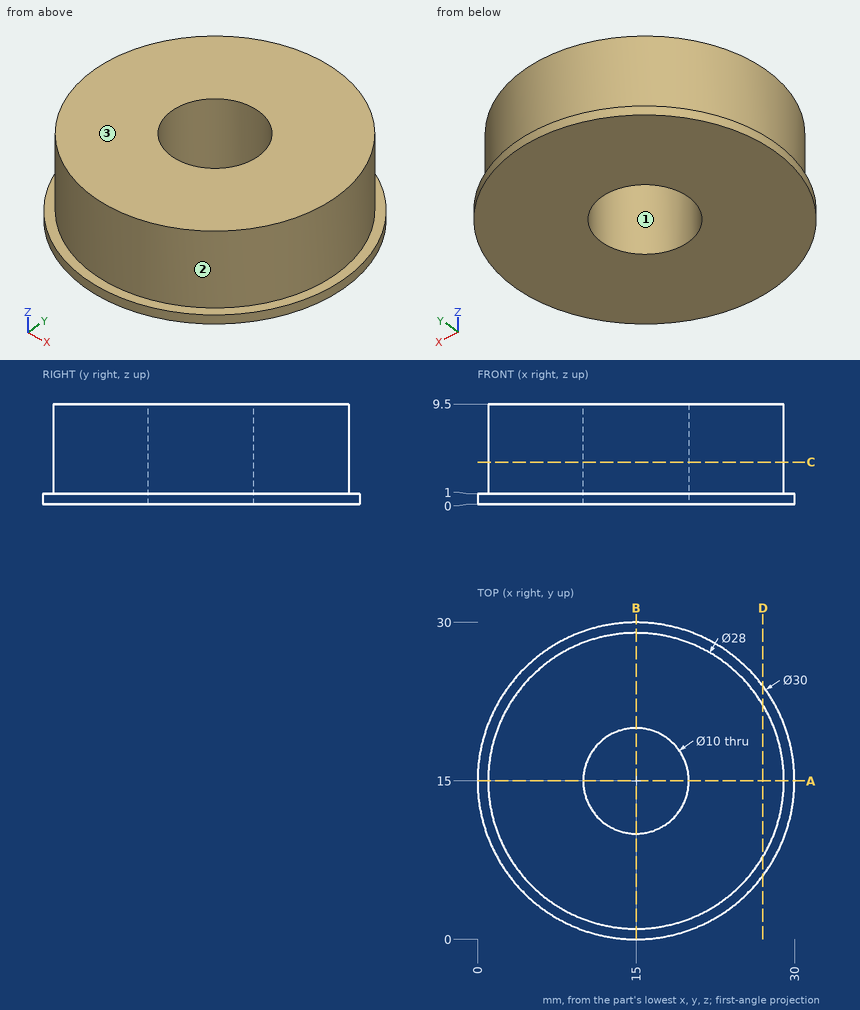
Geometry check sheet. Reference: drawing and pictorial views, mm from the part's lowest x, y, z. Coordinates: 2 decimals unless noted, no trailing zeros. Order: outer loops, then holes, each group sorted by start corner. A loop starts at its lowest first (then second) coordinate and runs counter-clockwise, first axis right, second up. Notation, with made-up numbers: (84.5, -38.5) -> (117.5, -38.5) arc R20 cw to (117.5, -32.5) -> close; hole circle Ø8 at (8.25, 50.25). An arc over 180 degrees is marked (long way). Write item = value, one per line. Start each with the question number.
1) Go/stop test with flat-tipped pins: P1, Ø2, axis at y = 8.5, z = 5.5, coming from the +X side; P2, Ø5, axis at x = 23.5, y = 16.5, coming from the -Z side; P3, Ø1, axis at x = 13.5, z = 2, coming from the +Y side; P4, Ø3, axis at y = 12.5, z = 5, coming from the -X side. Record where each tip stops, or that it passes through.
2) Mould release check, pull along X, two halves, no side actions. Record for the marked faces 1, 2 and 3: +X half, -X half, draft (parallel to the pull), parting line (faces both ways), or undercut.
3) Cross-section at A-A (y = 15). Enter the section's corners in (x, z), then the cut area to 3 significant figures.
4) Cross-section at C-C (z = 4). Enter the section's corners in (x, y).
5) Material ranges on L1, parallel to Y at x = 15, z = 4; L2, parallel to Y at x = 13.75, z = 7.75; L3, parallel to X at y = 17.75, z = 3, recorded low to high.
6) Cross-section at D-D (x = 27). Enter the section's corners in (y, z), then the cut area to 3 significant figures.
Ans:
q1.P1 = 27.87
q1.P2 = 0
q1.P3 = 28.96
q1.P4 = 1.04
q2.face_1 = undercut
q2.face_2 = parting line
q2.face_3 = draft
q3.outline = (0, 0) -> (10, 0) -> (10, 9.5) -> (1, 9.5) -> (1, 1) -> (0, 1) -> close; (20, 0) -> (30, 0) -> (30, 1) -> (29, 1) -> (29, 9.5) -> (20, 9.5) -> close
q3.area = 173 mm²
q4.outline = circle Ø28 at (15, 15); hole circle Ø10 at (15, 15)
q5.L1 = 1 to 10, 20 to 29
q5.L2 = 1.06 to 10.16, 19.84 to 28.94
q5.L3 = 1.27 to 10.82, 19.18 to 28.73
q6.outline = (6, 0) -> (24, 0) -> (24, 1) -> (22.21, 1) -> (22.21, 9.5) -> (7.79, 9.5) -> (7.79, 1) -> (6, 1) -> close
q6.area = 141 mm²
